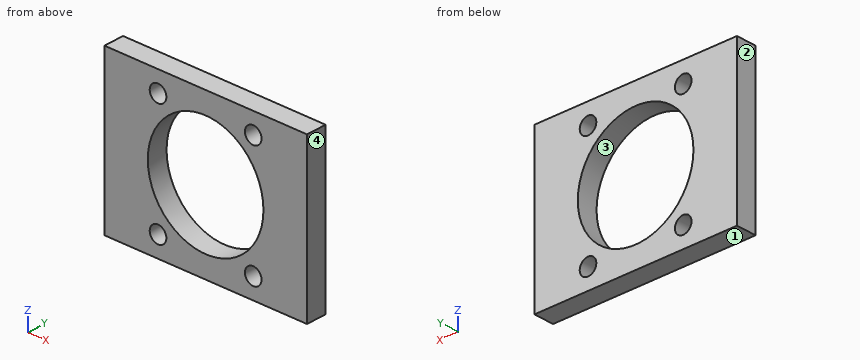
```python
from build123d import *

# Parameters (mm, degrees)
F0_W     = 33.5
F0_H     = 39
F0_R     = 2.05
F0_R_2   = 14.27
F1_DEPTH = 5
F2_W     = 8.25
F2_H     = 39
F3_DEPTH = 5


with BuildPart() as f1:
    # F0 (on Front) → F1 (new body)
    with BuildSketch(Plane.XZ):
        with Locations((-32.0278543325, -14.5)):
            Rectangle(F0_W, F0_H)
        with Locations((-43.7778543325, -29)):
            Circle(F0_R, mode=Mode.SUBTRACT)
        with Locations((-20.2778543325, -29)):
            Circle(F0_R, mode=Mode.SUBTRACT)
        with Locations((-43.7778543325, 0)):
            Circle(F0_R, mode=Mode.SUBTRACT)
        with Locations((-32.0278543325, -14.5)):
            Circle(F0_R_2, mode=Mode.SUBTRACT)
        with Locations((-20.2778543325, 0)):
            Circle(F0_R, mode=Mode.SUBTRACT)
    extrude(amount=F1_DEPTH)

    # F2 (on face) → F3 (join, through all)
    with BuildSketch(Plane.XZ.offset(5)):
        with Locations((-52.9028543325, -14.5)):
            Rectangle(F2_W, F2_H)
        with Locations((-11.1528543325, -14.5)):
            Rectangle(F2_W, F2_H)
    extrude(amount=-F3_DEPTH)


solid = f1.part
```
Work out the finished part from the listing and answer in its coordinate system (mm). Face numbers are marked on the shaded views. Give positions to 0.01 mm unless a question says otherwise; leave off trailing zeros. Loops run counter-clockwise (first coordinate to the right, second up) from the corner with the lowest first, then second, coordinate; pieces in that order, holes last. Notation, with made-up numbers: (-25.75, 14.25) -> (18.25, 14.25) arc R10 cw to (18.25, 23.25) -> close; hole circle Ø1 at (34, 68.5). An arc over 180 degrees is marked (long way). Write item = value, one per line. Start each with the question number.
(1) The mould has two halves that part along X. Classify the marked faces 1, 2, 3 and 4: +X half, -X half, draft (parallel to the pull), parting line (faces both ways), or undercut.
(2) Find section C-C on z = 1.5. Give the vertices of the cut face in (x, y), and give its area (3 significant figures).
(3) Find section B-B on y = -4.4. Give the vertices of the cut face in (x, z).
(4) Given pin 1 Ø3.5 at (x, z) = (-20.28, 0) entering from -Y, flat-ended and moving along its own axis, determine where the tip first touches the part or whether it passes through.
(5) Find section A-A on z = -14.5. Give the vertices of the cut face in (x, y), and give its area (3 significant figures).
(6) Find the intervals of material crossed by probe 1 along Z at (x, y) = (-32.5, -4.75); probe 2 along X at (y, z) = (-3.85, -9.5); probe 3 along X at (y, z) = (-3.5, -22.5), in increasing order. Write a range as from..to.
(7) Find section D-D on z = -9. Give the vertices of the cut face in (x, y), and give its area (3 significant figures).
From the geometry:
q1.face_1 = draft
q1.face_2 = -X half
q1.face_3 = undercut
q1.face_4 = +X half
q2.outline = (-57.03, -5) -> (-45.18, -5) -> (-45.18, 0) -> (-57.03, 0) -> close; (-42.38, -5) -> (-21.68, -5) -> (-21.68, 0) -> (-42.38, 0) -> close; (-18.88, -5) -> (-7.03, -5) -> (-7.03, 0) -> (-18.88, 0) -> close
q2.area = 222 mm^2
q3.outline = (-57.03, -34) -> (-7.03, -34) -> (-7.03, 5) -> (-57.03, 5) -> close; hole circle Ø28.54 at (-32.03, -14.5); hole circle Ø4.1 at (-43.78, -29); hole circle Ø4.1 at (-43.78, 0); hole circle Ø4.1 at (-20.28, -29); hole circle Ø4.1 at (-20.28, 0)
q4.pin_1 = through
q5.outline = (-57.03, -5) -> (-46.3, -5) -> (-46.3, 0) -> (-57.03, 0) -> close; (-17.76, -5) -> (-7.03, -5) -> (-7.03, 0) -> (-17.76, 0) -> close
q5.area = 107 mm^2
q6.probe_1 = -34..-28.76, -0.24..5
q6.probe_2 = -57.03..-45.39, -18.66..-7.03
q6.probe_3 = -57.03..-43.84, -20.21..-7.03
q7.outline = (-57.03, -5) -> (-45.2, -5) -> (-45.2, 0) -> (-57.03, 0) -> close; (-18.86, -5) -> (-7.03, -5) -> (-7.03, 0) -> (-18.86, 0) -> close
q7.area = 118 mm^2
